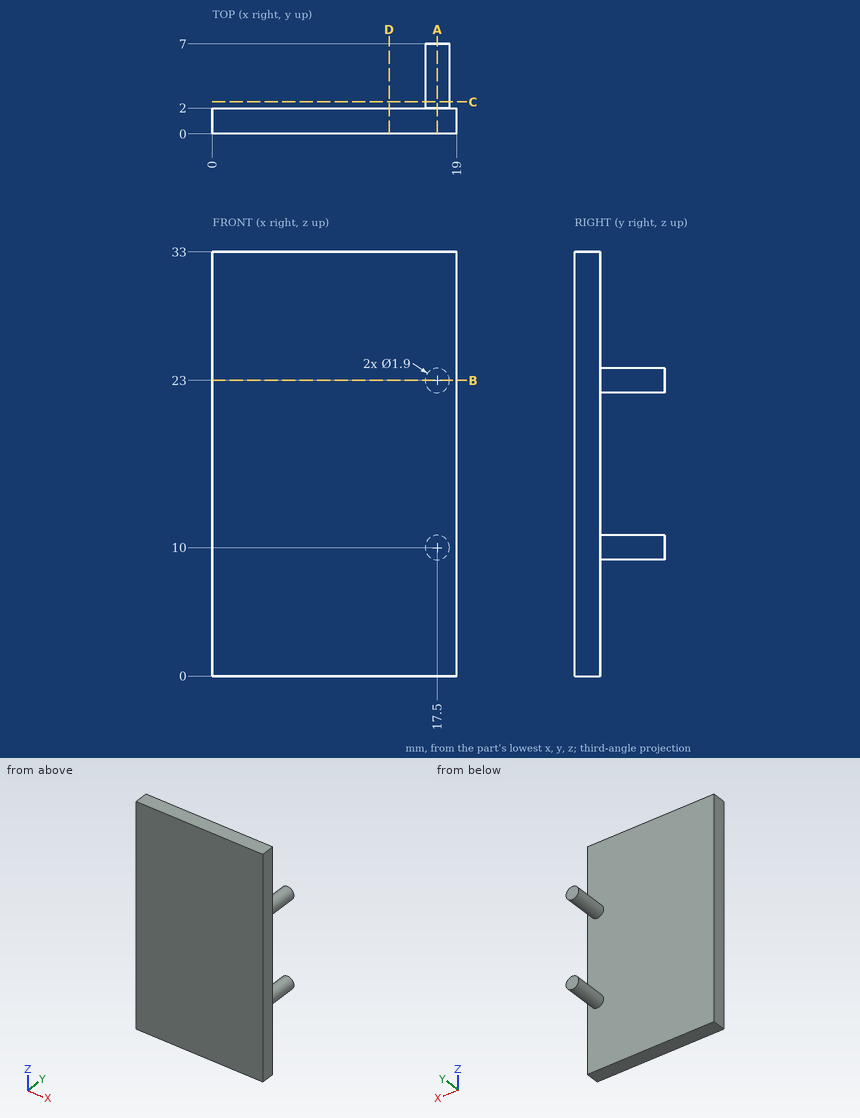
Part print with two shaded views. Sizes in mm from the minimum x, y, z corner. Coordinates: 2 decimals unless noted, no trailing zeros. Write each loop counter-clockwise with the first axis right and the second up, starting at its lowest first coordinate (ties: lowest second). Pieces come first, ordered by that corner, then holes.
1. Band-saw the part on D-D, the plane x = 13.75. Give the cut face in (y, z), and give its area (3 significant figures).
Answer block:
outline: (0, 0) - (2, 0) - (2, 33) - (0, 33) - close
area: 66.0 mm2
2. Band-saw the part on C-C, the plane y = 2.5. Give the cut face in (x, z).
Answer block:
outline: circle Ø1.9 at (17.5, 10); circle Ø1.9 at (17.5, 23)
3. Drop flat-ended pins along their axis: pin 1 (4 mm diameter, centred on x = 2, z = 9.5, fed in from -Y); pin 2 (5.5 mm diameter, centred on x = 7, z = 22.5, fed in from +Y); pin 3 (4 mm diameter, centred on x = 17, y = 6, fed in from +Z). Give the stop position or say it passes through.
Answer block:
pin 1: stops at y = 0
pin 2: stops at y = 2
pin 3: stops at z = 23.95
4. Band-saw the part on B-B, the plane z = 23. Give the cut face in (x, y).
Answer block:
outline: (0, 0) - (19, 0) - (19, 2) - (18.45, 2) - (18.45, 7) - (16.55, 7) - (16.55, 2) - (0, 2) - close
5. Band-saw the part on A-A, the plane x = 17.5. Give the cut face in (y, z), and give its area (3 significant figures).
Answer block:
outline: (0, 0) - (2, 0) - (2, 9.05) - (7, 9.05) - (7, 10.95) - (2, 10.95) - (2, 22.05) - (7, 22.05) - (7, 23.95) - (2, 23.95) - (2, 33) - (0, 33) - close
area: 85.0 mm2
6. Drill centre line: probe 1 along Y at (x, z) = (9.5, 10). Where is it in solid material? Low to high.
Answer block:
probe 1: y = 0 to 2
